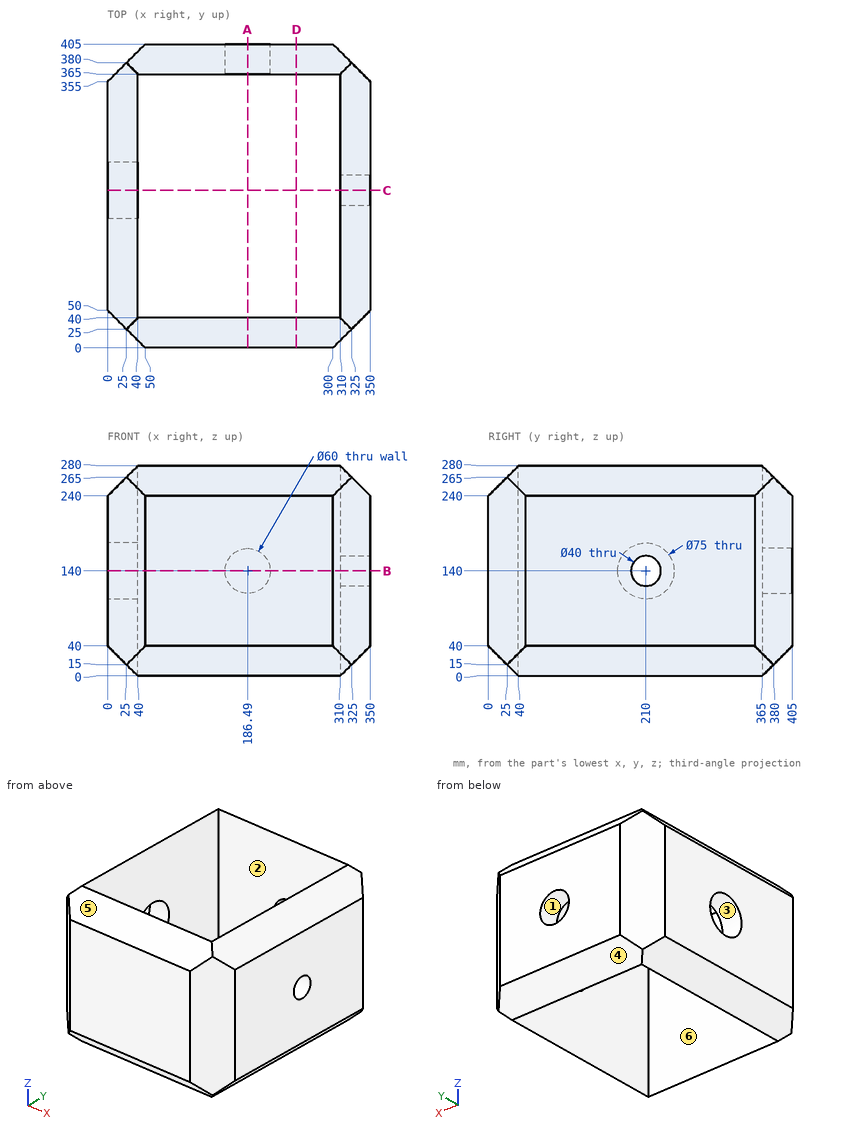
Input: dimensioned drawing with shaded views. Units: mm. Origin: part minimum x, y, z. A direction names the side the tool comes from. Coordinates: 2 decimals unless noted, no trailing zeros. Order: outer loops, then holes, each group sorted by start corner. A loop starts at its lowest first (then second) coordinate and runs counter-clockwise, first axis right, second up. Notation, with made-up numbers: M -2.75,-16.75 L 44.25,-16.75 A33 ccw 44.25,16.25 Z; hole C 14.25,21 d1. An arc over 180 degrees is marked long. Answer as CSV lines item,"result".
Q1. Section D-D on x = 251.5. Return the cut outline in (y, z).
Answers:
outline,"M 0,40 L 40,0 L 40,280 L 0,240 Z; M 365,0 L 405,40 L 405,240 L 365,280 Z"
Q2. First-contact query: P1, Ø1, axis at y = 43.5, z = 57.5, coming from the +X side; P2, Ø8, axis at x = 37.5, y = 333, coming from the -Z side. Flat tips, straight axial feed; report the tip coordinate or a pass-through.
Answers:
P1,"stops at x = 344"
P2,"stops at z = 0"
Q3. Line query: probe 1 along Y at (x, z) = (205, 97); probe 2 along X at (y, z) = (309.5, 185.5); probe 3 along X at (y, z) = (367.5, 157). Output: solid intervals per line, ascending. Write a range as [from, to].
Answers:
probe 1,"y = [0, 40], [365, 405]"
probe 2,"x = [0, 40], [310, 350]"
probe 3,"x = [12.5, 161.77], [211.21, 337.5]"
Q4. Set-up query: the marked faces 5 and 6. Return all of +Z, -Z, +X, -X, +Y, -Y with unobstructed straight access to the full face (end or side cutting, diameter ignored); none if empty.
Answers:
face 5,"+Z, +X, -X, -Y"
face 6,"+Z, -Z"
Q5. Section C-C on y = 210. Return the cut outline in (x, z).
Answers:
outline,"M 0,40 L 40,0 L 40,102.5 L 0,102.5 Z; M 0,177.5 L 40,177.5 L 40,280 L 0,240 Z; M 310,0 L 350,40 L 350,120 L 310,120 Z; M 310,160 L 350,160 L 350,240 L 310,280 Z"
Q6. Section A-A on x = 186.49. Return the cut outline in (y, z), and give its area (3 significant figures).
Answers:
outline,"M 0,40 L 40,0 L 40,280 L 0,240 Z; M 365,0 L 405,40 L 405,110 L 365,110 Z; M 365,170 L 405,170 L 405,240 L 365,280 Z"
area,"16,800 mm^2"
Q7. Draft query along Z for the marked faces 1, 2, 3 and 4. Return one class per face: pulls with the +Z half, pulls with the -Z half, needs draft (parallel to the pull), parting line crosses it, or undercut.
Answers:
face 1,"undercut"
face 2,"needs draft"
face 3,"undercut"
face 4,"pulls with the -Z half"
Q8. Section B-B on z = 140. Return the cut outline in (x, y).
Answers:
outline,"M 0,50 L 50,0 L 300,0 L 350,50 L 350,190 L 310,190 L 310,40 L 40,40 L 40,172.5 L 0,172.5 Z; M 0,247.5 L 40,247.5 L 40,365 L 156.49,365 L 156.49,405 L 50,405 L 0,355 Z; M 216.49,365 L 310,365 L 310,230 L 350,230 L 350,355 L 300,405 L 216.49,405 Z"
